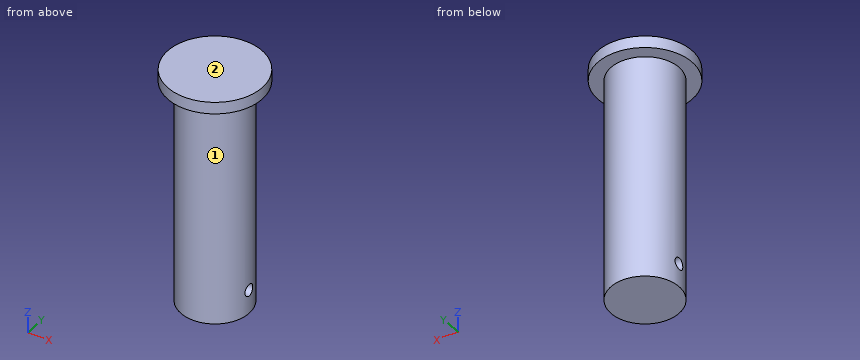
from build123d import *

# Parameters (mm, degrees)
SKETCH_1_R               = 14.44
EXTRUDE_1_DEPTH          = 100
SKETCH_3_R               = 20
EXTRUDE_3_DEPTH          = 5
CUT_EXTRUDE_1_DEPTH      = 104.923048454
CUT_EXTRUDE_1_DEPTH_BACK = 104.923048454
SKETCH_4_R               = 2.5


with BuildPart() as part:
    # 草图1 → 凸台-拉伸1 (new body)
    with BuildSketch(Plane.XY):
        Circle(SKETCH_1_R)
    extrude(amount=EXTRUDE_1_DEPTH)

    # 草图3 → 凸台-拉伸3 (add)
    with BuildSketch(Plane.XY.offset(100)):
        Circle(SKETCH_3_R)
    extrude(amount=-EXTRUDE_3_DEPTH)

    # 草图4 → 切除-拉伸1 (cut, two sides: drawn at the far end of the back side and taken through both)
    with BuildSketch(Plane(origin=(0, 0, 0), x_dir=(0, 0, -1), z_dir=(1, 0, 0)).offset(-CUT_EXTRUDE_1_DEPTH_BACK)):
        with Locations(Location((-10, 0, 0), (0, 0, 180))):
            Circle(SKETCH_4_R)
    extrude(amount=CUT_EXTRUDE_1_DEPTH + CUT_EXTRUDE_1_DEPTH_BACK, mode=Mode.SUBTRACT)


solid = part.part
Work out the finished part from the listing and answer in its coordinate system (mm). Face numbers are marked on the shaded views. A direction names the side the tool comes from. Round coordinates to 2 decimals unless told otherwise and drop trailing zeros. Loops run counter-clockwise (first coordinate to the right, second up) from the corner with the lowest first, then second, coordinate; pieces in that order, holes last. Notation, with made-up numbers: (38.25, -8) -> (81.25, -8) arc R7 cw to (81.25, 5) -> close; hole circle Ø10 at (-3, 15.25). An arc over 180 degrees is marked (long way). Use one line per item in the form item = value.
(1) Flat-ended cylindrical pins translate along their axes: P1, Ø12, axis at y = 7.5, z = 80, coming from the -X side; P2, Ø8, axis at x = -14.5, z = 35.5, coming from the +Y side; P3, Ø5, axis at x = 4.5, z = 53.5, coming from the +Y side; P4, Ø4.5, axis at y = 0, z = 10, coming from the +X side. Find the tip coordinate at first contact, or state that the pin passes through.
Answer list:
P1 = -14.36
P2 = 9.91
P3 = 14.3
P4 = through
(2) Find section A-A on y = 0. Give the vertices of the cut face in (x, z).
Answer list:
outline = (-20, 95) -> (-14.44, 95) -> (-14.44, 12.5) -> (14.44, 12.5) -> (14.44, 95) -> (20, 95) -> (20, 100) -> (-20, 100) -> close; (-14.44, 0) -> (14.44, 0) -> (14.44, 7.5) -> (-14.44, 7.5) -> close
(3) Find section C-C on z = 58. Give the vertices of the cut face in (x, y), then the cut area to 3 significant figures.
Answer list:
outline = circle Ø28.88 at (0, 0)
area = 655 mm2
(4) Find section B-B on x = 0. Give the vertices of the cut face in (y, z).
Answer list:
outline = (-20, 95) -> (-14.44, 95) -> (-14.44, 0) -> (14.44, 0) -> (14.44, 95) -> (20, 95) -> (20, 100) -> (-20, 100) -> close; hole circle Ø5 at (0, 10)
(5) Straight lines are drawn through the part: line 1 (Z direction, x = -14, y = -13.5); line 2 (Y direction, x = 2, z = 10); line 3 (Y direction, x = 8.5, z = 10). For each, find the intervals that lie inside material, in ascending order.
Answer list:
line_1 = 95 to 100
line_2 = -14.3 to -2.5, 2.5 to 14.3
line_3 = -11.67 to -2.5, 2.5 to 11.67
(6) Find section D-D on y = -8. Give the vertices of the cut face in (x, z), then the cut area to 3 significant figures.
Answer list:
outline = (-18.33, 95) -> (-12.02, 95) -> (-12.02, 0) -> (12.02, 0) -> (12.02, 95) -> (18.33, 95) -> (18.33, 100) -> (-18.33, 100) -> close
area = 2,470 mm2
(7) A tool of negligible diameter and unlimited length cuts with its end or side. For the marked faces 1 and 2, from which of +Z, -Z, +X, -X, +Y, -Y can it reach the whole face along a straight path? Write none if from no direction.
Answer list:
face_1 = -Z
face_2 = +Z, +X, -X, +Y, -Y
